Autodesk Inventor part; units mm, degrees
ref_plane "YZ Plane" through (0, 0, 0) normal (1, 0, 0) x (0, 1, 0)
ref_plane "XZ Plane" through (0, 0, 0) normal (0, 1, 0) x (-1, 0, 0)
ref_plane "XY Plane" through (0, 0, 0) normal (0, 0, 1) x (1, 0, 0)
sketch "Sketch1" plane through (0, 0, 0) normal (0, 0, 1) x (1, 0, 0)
  circle A0 centre (0, 0) radius 12.5
  circle A1 centre (0, 0) radius 5
  dimension "d0" = 25
  dimension "d1" = 10
extrude "Extrusion1" add sketch "Sketch1" along normal blind 15
sketch "Sketch2" plane through (0, 0, 15) normal (0, 0, 1) x (1, 0, 0)
  circle A0 centre (0, 0) radius 17.5
  dimension "d4" = 35
extrude "Extrusion2" add sketch "Sketch2" along normal blind 5
sketch "Sketch3" plane through (0, 0, 20) normal (0, 0, 1) x (1, 0, 0)
  circle A0 centre (0, 0) radius 5
  dimension "d7" = 10
extrude "Extrusion3" cut sketch "Sketch3" against normal through all
sketch "Sketch5" plane through (0, 0, 0) normal (0, 0, -1) x (-1, 0, 0)
  circle A0 centre (0, 8.75) radius 2
  circle A1 centre (-7.5777, -4.375) radius 2
  circle A2 centre (7.5777, -4.375) radius 2
  point P0 (0, 0)
  dimension "d10" = 4
  dimension "d11" = 8.75
  dimension "d14" = 360
extrude "Extrusion4" cut sketch "Sketch5" against normal through all
thread "Thread1"
thread "Thread2"
thread "Thread3"
properties part number "CP013" material "ABS Plastic"
Read the model definition and answer for the solid it produces. Units are mm, in the model's axes. A direction names the side the tool comes from. Give positions to 0.01 mm unless a question says otherwise; leave off trailing zeros. Order: outer loops, then holes, each group sorted by start corner. A loop starts at its lowest first (then second) coordinate and runs counter-clockwise, first axis right, second up. Notation, with made-up numbers: (72.5, 20.25) -> (109.5, 20.25) arc R29 ccw to (109.5, 55.25) -> close; hole circle Ø1 at (59, -38.75). An arc over 180 degrees is marked (long way). Write item = value, one per line.
1. For faces 1 (the face through (11, -8, 15)), 2 (the face through (-0.2, -5.4, 0)), determine the directions among +Z, -Z, +X, -X, +Y, -Y from which every point of the face is accessible in a straight line to the end or side of a thin tool.
Numbers:
face_1 = -Z
face_2 = -Z, +X, -X, +Y, -Y
2. Given pin 1 (1.5 mm diameter, centred on x = -5.5, y = 14, fed in from -Z); pin 2 (1 mm diameter, centred on x = 9, z = 7, fed in from +Y); pin 3 (1.5 mm diameter, centred on x = 5.5, z = 5.5, fed in from +Y), each flat-ended and moving along its own axis, determine where each tip first touches the part or whether it passes through.
Numbers:
pin_1 = 15
pin_2 = 9.17
pin_3 = 11.56
3. A cutting plane is placed at A-A, the plane y = 0. Write down the section's boundary in (x, z), and give its area (3 significant figures).
Numbers:
outline = (-17.5, 15) -> (-12.5, 15) -> (-12.5, 0) -> (-5, 0) -> (-5, 20) -> (-17.5, 20) -> close; (5, 0) -> (12.5, 0) -> (12.5, 15) -> (17.5, 15) -> (17.5, 20) -> (5, 20) -> close
area = 350 mm²
4. A cutting plane is placed at B-B, the plane x = 0. Write down the section's boundary in (y, z).
Numbers:
outline = (-17.5, 15) -> (-12.5, 15) -> (-12.5, 0) -> (-5, 0) -> (-5, 20) -> (-17.5, 20) -> close; (5, 0) -> (6.75, 0) -> (6.75, 20) -> (5, 20) -> close; (10.75, 0) -> (12.5, 0) -> (12.5, 15) -> (17.5, 15) -> (17.5, 20) -> (10.75, 20) -> close
5. A cutting plane is placed at C-C, the plane x = -4. Write down the section's boundary in (y, z).
Numbers:
outline = (-17.04, 15) -> (-11.84, 15) -> (-11.84, 0) -> (-3, 0) -> (-3, 20) -> (-17.04, 20) -> close; (3, 0) -> (11.84, 0) -> (11.84, 15) -> (17.04, 15) -> (17.04, 20) -> (3, 20) -> close
6. A cutting plane is placed at D-D, the plane z = 9.5. Write down the section's boundary in (x, y) (3 decimals), and give its area (3 significant figures).
Numbers:
outline = circle Ø25 at (0, 0); hole circle Ø4 at (-7.578, -4.375); hole circle Ø10 at (0, 0); hole circle Ø4 at (0, 8.75); hole circle Ø4 at (7.578, -4.375)
area = 375 mm²
7. The mould has two halves that part along Y. Classify faces 3 (the face through (-1.08, -4.88, 10.14)), 4 (the face through (-8.5, -6.15, 9.86)), 5 (the face through (-13.887, 10.648, 17.465)), 6 (the face through (4, -4, 20)): +Y half, -Y half, draft (parallel to the pull), parting line (faces both ways), or undercut.
Numbers:
face_3 = undercut
face_4 = undercut
face_5 = parting line
face_6 = draft
8. Straight lines are drawn through the part: line 1 along Y through (x, z) = (0, 18.75); line 2 along Y through (x, z) = (0, 8); line 3 along X through (y, z) = (-4.5, 3.75). For each, find the intervals that lie inside material, in ascending order.
Numbers:
line_1 = -17.5 to -5, 5 to 6.75, 10.75 to 17.5
line_2 = -12.5 to -5, 5 to 6.75, 10.75 to 12.5
line_3 = -11.66 to -9.57, -5.58 to -2.18, 2.18 to 5.58, 9.57 to 11.66
